Geometry: see drawing. Coordinates: mm, zero at the bounding-box minimum. A direction names the side the tool comes from. Round coordinates to 2 decimals unless told otherwise and drop trailing zeros. Order: outer loops, then holes, each group sorted by start corner. A loop starts at its lowest first (then second) coordinate and runs counter-clockwise, first axis right, second up. Notation, with made-up numbers: (88, 38) - (98, 38) arc R9 cw to (98, 54) - close; hole circle Ø3 at (64.5, 37.25). An arc over 180 degrees is marked (long way). Put each result on its own line as item: value. Start each with the question number.
1) Section C-C on y = 4.1. State how many separate pieces and enclosed holes the cut face has, then the cut area to 3 significant figures.
2) Mould query, pull axis Z, two halves, no side actions, for the marked faces 6, 7 and 8. Classes: +Z half, -Z half, draft (parallel to the pull), parting line (faces both ways), or undercut.
3) Access query for the marked faces 1, 2, 3, 4 and 5. Directions: +Z, -Z, +X, -X, +Y, -Y. A direction counts if a zero-diameter tool reaches every point of the face in a straight line with its end or side. Return the directions, or none.
4) Line query: probe 1 along X at (y, z) = (1.7, 43.75); probe 2 along Z at (x, y) = (9, 1.75); probe 3 along X at (y, z) = (3.45, 45). Output: solid intervals per line, ascending. Write a range as [from, to].
5) Contact query for flat-ended pins moving along their axis: P1, Ø1.5, axis at y = 2.5, z = 8.5, coming from the -X side; P2, Ø2, axis at x = 11, y = 2.5, coming from the +Z side; P3, Ø3, axis at x = 30.5, y = 1.5, coming from the -Z side; P4, Ø1.2, axis at y = 3.5, z = 14, coming from the +X side. Output: stop coordinate, or through.
6) Section B-B on x = 3. Output: boundary loops of the cut face in (y, z).
7) Section A-A on z = 36.25. Output: boundary loops of the cut face in (x, y).
8) Section D-D on z = 11.5. Output: boundary loops of the cut face in (x, y).
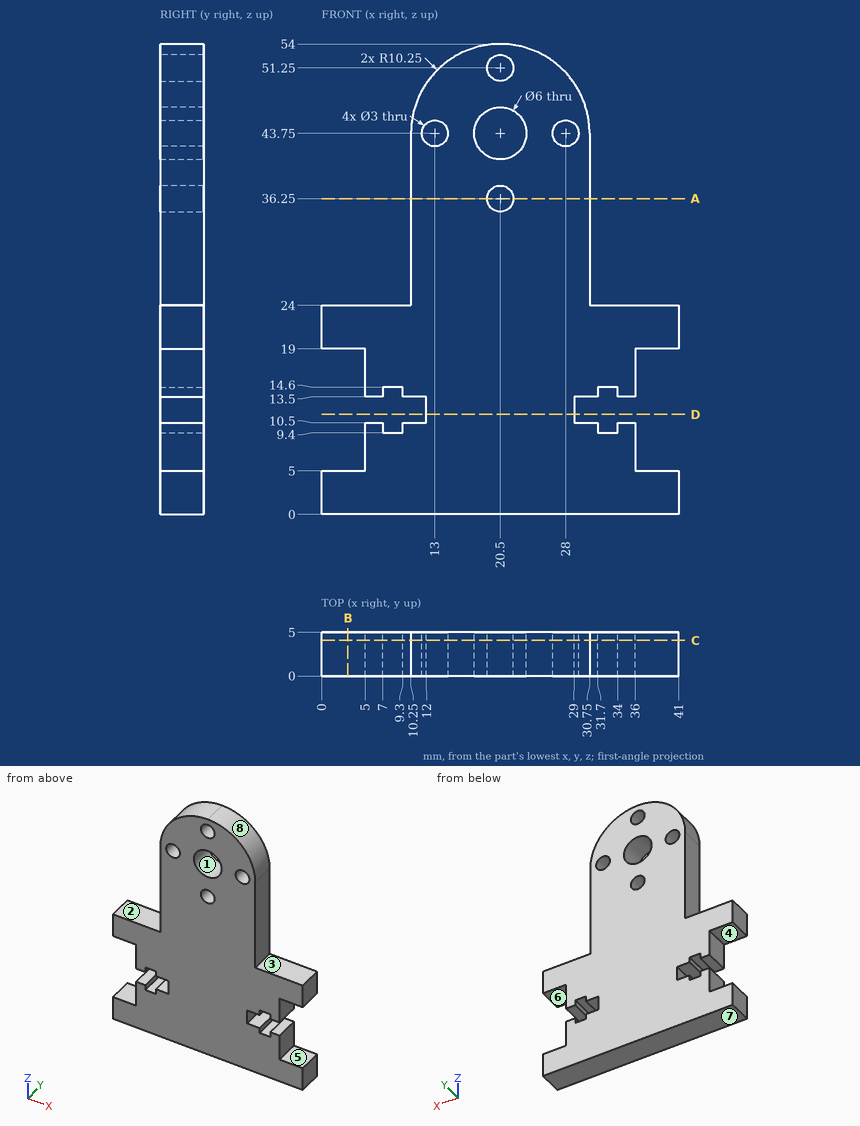
Answer sheet:
1. separate pieces: 1
1. enclosed holes: 5
1. area: 1,310 mm^2
2. face 6: undercut
2. face 7: -Z half
2. face 8: +Z half
3. face 1: +Y, -Y
3. face 2: +Z, -X, +Y, -Y
3. face 3: +Z, +X, +Y, -Y
3. face 4: -X, +Y, -Y
3. face 5: +X, +Y, -Y
4. probe 1: [10.25, 11.5], [14.5, 17.5], [23.5, 26.5], [29.5, 30.75]
4. probe 2: [0, 9.4], [14.6, 24]
4. probe 3: [10.33, 12.17], [13.83, 17.77], [23.23, 27.17], [28.83, 30.67]
5. P1: x = 5
5. P2: z = 49.48
5. P3: z = 0
5. P4: x = 36
6. outline: (0, 0) - (5, 0) - (5, 5) - (0, 5) - close; (0, 19) - (5, 19) - (5, 24) - (0, 24) - close
7. outline: (10.25, 0) - (19, 0) - (19, 5) - (10.25, 5) - close; (22, 0) - (30.75, 0) - (30.75, 5) - (22, 5) - close
8. outline: (12, 0) - (29, 0) - (29, 5) - (12, 5) - close
